```python
from build123d import *

# Parameters (mm, degrees)
SKETCH1_R                              = 7.1
PISTON_DEPTH                           = 5
SKETCH2_R                              = 3.175
ROD_DEPTH                              = 25.614
F_056_8_32_INTERNAL_THREAD_D           = 3.4544
F_056_8_32_INTERNAL_THREAD_DEPTH       = 14.07744
F_056_8_32_INTERNAL_THREAD_CBORE_D     = 4.1656
F_056_8_32_INTERNAL_THREAD_CBORE_DEPTH = 11.684
F_056_8_32_INTERNAL_THREAD_TIP         = 1.037806461
ROD_END_CHAMFER_SIZE                   = 0.3
WRENCH_FLATS_DEPTH                     = 28.511761049
WRENCH_FLATS_DEPTH_BACK                = 28.511761049


with BuildPart() as part:
    # Sketch1 → Piston (new body)
    with BuildSketch(Plane.XY):
        Circle(SKETCH1_R)
    extrude(amount=PISTON_DEPTH)

    # Sketch2 → Rod (add)
    with BuildSketch(Plane(origin=(0, 0, 0), x_dir=(-1, 0, 0), z_dir=(0, 0, -1))):
        with Locations(Location((0, 0, 0), (0, 0, 90))):
            Circle(SKETCH2_R)
    extrude(amount=-ROD_DEPTH)

    # 056 #8-32 Internal Thread
    with Locations(Plane(origin=(0, 0, 25.614), x_dir=(0, 1, 0), z_dir=(0, 0, 1))):
        with Locations((0, 0)):
            CounterBoreHole(F_056_8_32_INTERNAL_THREAD_D / 2, F_056_8_32_INTERNAL_THREAD_CBORE_D / 2, F_056_8_32_INTERNAL_THREAD_CBORE_DEPTH, depth=F_056_8_32_INTERNAL_THREAD_DEPTH)
            with Locations((0, 0, -(F_056_8_32_INTERNAL_THREAD_DEPTH + F_056_8_32_INTERNAL_THREAD_TIP / 2))):  # 118° drill point
                Cone(0, F_056_8_32_INTERNAL_THREAD_D / 2, F_056_8_32_INTERNAL_THREAD_TIP, mode=Mode.SUBTRACT)

    # Rod End Chamfer
    rod_end_chamfer_edges = [part.edges().sort_by_distance(p)[0] for p in [
        (0, -2.0828, 25.614),
        (0, -3.175, 25.614),
    ]]
    chamfer(rod_end_chamfer_edges, length=ROD_END_CHAMFER_SIZE)

    # Sketch11 → Wrench Flats (cut, two sides: drawn at the far end of the back side and taken through both)
    with BuildSketch(Plane(origin=(0, 0, 0), x_dir=(1, 0, 0), z_dir=(0, 1, 0)).offset(-WRENCH_FLATS_DEPTH_BACK)):
        Polygon((-2.8, -25.614), (-2.8, -22.614), (-7.8, -19.727248654), (-7.8, -25.614), align=None)
        Polygon((2.8, -25.614), (2.8, -22.614), (7.8, -19.727248654), (7.8, -25.614), align=None)
    extrude(amount=WRENCH_FLATS_DEPTH + WRENCH_FLATS_DEPTH_BACK, mode=Mode.SUBTRACT)


solid = part.part
```
The listing builds one solid part. Answer for the finished solid, in the listing's coordinates (mm). A direction names the side the tool comes from. Coordinates: 2 decimals unless noted, no trailing zeros. Write each loop counter-clockwise with the first axis right and the second up, starting at its lowest first coordinate (ties: lowest second). Pieces come first, ordered by that corner, then holes.
Q1. Which of the six approach directions +Z, -Z, +X, -X, +Y, -Y give full straight-line access (tool end or side, diameter ignored) to faces 1 (the flat face through (3.1, -1.5, 5)), 2 (the flat face through (-2.8, 0, 24)), 3 (the flat face through (2.8, 0, 24)), 4 (the conical face through (-0.06, 2.99, 25.5)), 5 (the conical face through (0.06, -2.99, 25.5))?
Returned:
face 1: +Z
face 2: +Z, -X, +Y, -Y
face 3: +Z, +X, +Y, -Y
face 4: +Z, +Y
face 5: +Z, -Y
Q2. Section B-B, the plane z = 12 is taken. Write down the section's boundary in (x, y) (3 decimals).
Returned:
outline: circle Ø6.35 at (0, 0); hole circle Ø3.454 at (0, 0)
Q3. The mould has two halves that part along X. Classify faces 6 (the cylindrical face through (3.15, -0.41, 15.01)), 7 (the conical face through (0.27, 0.14, 10.68)), 8 (the flat face through (0, 0, 0)): released by +X, released by -X, zero draft, split by the parting line, or undercut.
Returned:
face 6: split by the parting line
face 7: undercut
face 8: zero draft
Q4. Section C-C, the plane y = -6 is taken. Write down the section's boundary in (x, z).
Returned:
outline: (-3.8, 0) - (3.8, 0) - (3.8, 5) - (-3.8, 5) - close
Q5. Find the intervals of material crossed by line 1 along X through (y, z) = (0, 23); line 2 along X through (y, z) = (0, 13.1) (3 decimals); line 3 along Y through (x, z) = (0, 21) (3 decimals), in increasing order.
Returned:
line 1: x = -2.8 to -2.08, 2.08 to 2.8
line 2: x = -3.175 to -1.727, 1.727 to 3.175
line 3: y = -3.175 to -2.083, 2.083 to 3.175
Q6. Given P1, Ø1, axis at x = -4.5, y = -1, coming from the +Z side; P2, Ø1.2, axis at x = -0.5, y = 0.5, coming from the +Z side; P3, Ø3.5, axis at y = -0.5, z = 24.5, coming from the -X side, each flat-ended and moving along its own axis, determine where each tip first touches the part or whether it passes through.
Returned:
P1: stops at z = 5
P2: stops at z = 11.28
P3: stops at x = -2.8
Q7. Section A-A, the plane z = 6.75 is taken. Write down the section's boundary in (x, y) (3 decimals), then the cut area to 3 significant figures.
Returned:
outline: circle Ø6.35 at (0, 0)
area: 31.7 mm2
Q8. Section D-D, the plane x = -4.25 is taken. Write down the section's boundary in (y, z).
Returned:
outline: (-5.69, 0) - (5.69, 0) - (5.69, 5) - (-5.69, 5) - close
